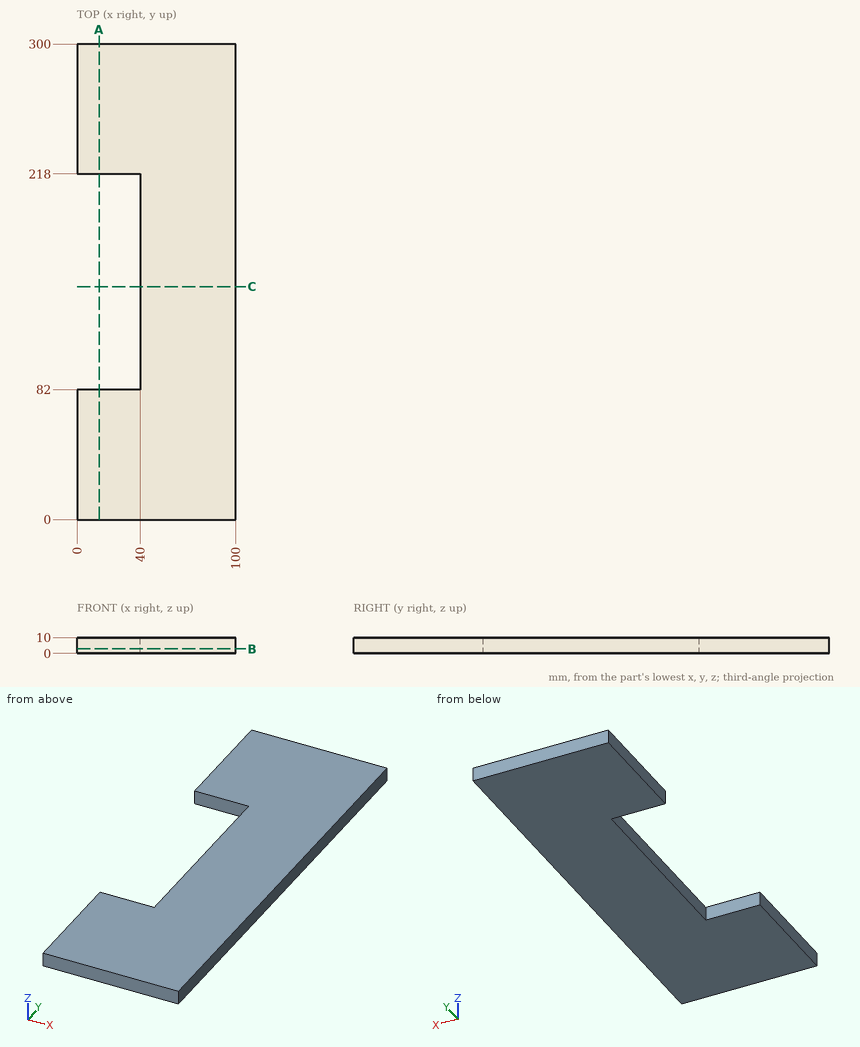
Source: three-view drawing plus pictorial views. Frame: mm from the lowest corner of the part. Give positions to 0.01 mm unless a question says otherwise; leave off trailing zeros. Write each loop counter-clockwise with the first axis right and the second up, starting at its lowest first coordinate (ties: lowest second). Pieces come first, ordered by that corner, then holes. Notation, with made-up numbers: (-7.5, -2.5) -> (10.5, -2.5) arc R33 cw to (10.5, 27.5) -> close; hole circle Ø7 at (69, 83.5). An arc over 180 degrees is marked (long way). Answer in a Markdown table with one row per item.
(1) Section query B-B on z = 2.75. Return loops of the section in (x, y), then the cut area to 3 significant figures.
Answers below:
| item | result |
|---|---|
| outline | (0, 0) -> (100, 0) -> (100, 300) -> (0, 300) -> (0, 218) -> (40, 218) -> (40, 82) -> (0, 82) -> close |
| area | 24,600 mm^2 |
(2) Section query C-C on y = 147. Return loops of the section in (x, z), then the cut area to 3 significant figures.
Answers below:
| item | result |
|---|---|
| outline | (40, 0) -> (100, 0) -> (100, 10) -> (40, 10) -> close |
| area | 600 mm^2 |
(3) Section query A-A on x = 14. Return loops of the section in (y, z).
Answers below:
| item | result |
|---|---|
| outline | (0, 0) -> (82, 0) -> (82, 10) -> (0, 10) -> close; (218, 0) -> (300, 0) -> (300, 10) -> (218, 10) -> close |
(4) Ray query, line 1 along Y through (x, z) = (23.5, 7.25); line 2 along X through (y, z) = (189, 7.5). Return the intervals inside material, ascending. Write a range as [from, to].
Answers below:
| item | result |
|---|---|
| line 1 | [0, 82], [218, 300] |
| line 2 | [40, 100] |
(5) Pin query (flat end, axial travel): pin 1 (3 mm diameter, centred on y = 162, z = 3.5, fed in from -X). Return the tip coordinate at first contact, or that it passes through.
Answers below:
| item | result |
|---|---|
| pin 1 | x = 40 |
